Design review of the part built by this model. Coordinates are the model's own, in mm. Give positions to 0.01 mm unless a question says otherwise; leave off trailing zeros. Loops run counter-clockwise (first coordinate to the right, second up) from the corner with the lowest first, then second, coordinate; pieces in that order, holes last. Notation, with made-up numbers: (6, 52.25) -> (14, 52.25) arc R20 ccw to (14, 76.25) -> close; hole circle Ø11 at (83.5, 57). An arc over 180 degrees is marked (long way). Use CSV: the item, a comma, the result in double quotes. Start each with the question number.
Item 1: We need section B-B (x = 25). State the section outline as (y, z) points, plus the area to 3 significant figures.
Item 2: The part is to be moulded in two halves that separate along Z. For faces 1 (the face through (25.751, 1.521, -102.615)), 2 (the face through (79, 3, -107)), say which applies: +Z half, -Z half, draft (parallel to the pull), parting line (faces both ways), or undercut.
Item 3: Wall thickness on line 1 along Z through (x, y) = (185, 1.5); line 2 along X through (y, z) = (0.7, -25): over which ranges is each line inside the solid? List them lowest first. Write a range as from..to.
Item 4: We need section A-A (z = -25). State the section outline as (x, y) points.
Item 5: Clearance check with flat-ended pins moving along their axes: pin 1 (0.9 mm diameter, centred on y = 1.5, z = 2.5, fed in from +X); pin 2 (1.5 mm diameter, centred on x = -2, y = 1.5, fed in from -Z). State where each tip first meets the part, or that it passes through.
from build123d import *

# Parameters (mm, degrees)
BOSS_EXTRUDE1_DEPTH  = 3
SKETCH2_R            = 2.5
CUT_EXTRUDE1_DEPTH   = 305.070715459
LPATTERN1_COUNT      = 3
LPATTERN1_PITCH      = 80
LPATTERN1_COUNT_DIR2 = 3
LPATTERN1_PITCH_DIR2 = 80


with BuildPart() as part:
    # Sketch1 → Boss-Extrude1 (new body)
    with BuildSketch(Plane(origin=(0, 0, 0), x_dir=(1, 0, 0), z_dir=(0, 1, 0))):
        Polygon((0, -5), (210, -5), (210, 0), (215, 0), (215, 210), (210, 210), (210, 215), (0, 215), (0, 210), (-5, 210), (-5, 0), (0, 0), align=None)
    extrude(amount=BOSS_EXTRUDE1_DEPTH)

    # Sketch2 → Cut-Extrude1 (cut, through all)
    with BuildSketch(Plane(origin=(0, 3, 0), x_dir=(1, 0, 0), z_dir=(0, 1, 0))):
        with Locations(Location((25, 25, 0), (0, 0, 270))):
            Circle(SKETCH2_R)
    cut_extrude1 = extrude(amount=-CUT_EXTRUDE1_DEPTH, mode=Mode.SUBTRACT)

    # LPattern1: Cut-Extrude1 3 × 3
    with Locations(*[(i * LPATTERN1_PITCH, 0, -j * LPATTERN1_PITCH_DIR2) for i in range(LPATTERN1_COUNT) for j in range(LPATTERN1_COUNT_DIR2) if (i, j) != (0, 0)]):
        add(cut_extrude1, mode=Mode.SUBTRACT)


solid = part.part
Results found:
1,outline,"(0, -215) -> (3, -215) -> (3, -187.5) -> (0, -187.5) -> close; (0, -182.5) -> (3, -182.5) -> (3, -107.5) -> (0, -107.5) -> close; (0, -102.5) -> (3, -102.5) -> (3, -27.5) -> (0, -27.5) -> close; (0, -22.5) -> (3, -22.5) -> (3, 5) -> (0, 5) -> close"
1,area,"615 mm²"
2,face 1,"undercut"
2,face 2,"draft"
3,line 1,"-215..-187.5, -182.5..-107.5, -102.5..-27.5, -22.5..5"
3,line 2,"-5..22.5, 27.5..102.5, 107.5..182.5, 187.5..215"
4,outline,"(-5, 0) -> (22.5, 0) -> (22.5, 3) -> (-5, 3) -> close; (27.5, 0) -> (102.5, 0) -> (102.5, 3) -> (27.5, 3) -> close; (107.5, 0) -> (182.5, 0) -> (182.5, 3) -> (107.5, 3) -> close; (187.5, 0) -> (215, 0) -> (215, 3) -> (187.5, 3) -> close"
5,pin 1,"x = 210"
5,pin 2,"z = -210"
